Read the model definition and answer for the solid it produces. Units are mm, in the model's axes. A direction names the side the tool comes from. Coordinates: 2 decimals unless noted, no trailing zeros. Loops run counter-clockwise (first coordinate to the right, second up) from the corner with the lowest first, then second, coordinate; pieces in that order, holes last. Notation, with made-up numbers: M 29,31.25 L 83,31.25 A23 cw 83,49.25 Z; hole C 20.5,-28 d2. An arc over 180 degrees is marked long. Use one line per item in the form item = value. Start each with the question number.
1. The part is cut by section A-A (z = -20). Give the vertices of the cut face in (x, y).
2. For a pull along X with two mould halves and no side action, classify faces 1 (the conical face through (-86.28, -1.239, -12.833)), 2 (the conical face through (-65.93, 5.98, -7.72)), 3 (the flat face through (-58, 0, -40.287)) as released by +X, released by -X, zero draft, split by the parting line, or undercut.
3. Flat-ended cylindrical pins translate along their axes: pin 1 (12 mm diameter, centred on x = -53.5, y = 44.5, fed in from +Z); pin 2 (5 mm diameter, centred on y = -13.5, z = 14.5, fed in from +X); pin 3 (3 mm diameter, centred on x = -44, z = -13.5, fed in from -Y). Find the tip coordinate at first contact, or state that the pin passes through.
4. Find the intervals of material crossed by probe 1 along X at (y, z) = (-36.5, 19); probe 2 along X at (y, z) = (-6, 21.5); probe 3 along Y at (x, z) = (-81, 21), in increasing order. Write a range as [from, to].
5. The part is cut by section B-B (z = 21.5). Give the vertices of the cut face in (x, y).
6. A tool of negligible diameter and unlimited length cuts with its end or side. For faces 4 (the cylindrical face through (-83.5, -1.12, -27.41)), 5 (the conical face through (-107.31, 37.72, 29.41)), from which of +Z, -Z, +X, -X, +Y, -Y can it reach the whole face along a straight path? Write none if from no direction.
7. The part is cut by section C-C (z = 13). Give the vertices of the cut face in (x, y), plus the area to 3 significant figures.
from build123d import *

# Parameters (mm, degrees)
F2_R     = 25.4
F3_DEPTH = 25.4
F4_DEPTH = 76.2


with BuildPart() as f1:
    # F0 (on Front) → F1 (revolve)
    with BuildSketch(Plane.XZ):
        Polygon((-58.1262356877, -14.8871221304), (-58.1262356877, -40.2871221304), (-32.7262356877, -40.2871221304), (-32.7262356877, -14.8871221304), (11.7363044992, 17.9430041462), (3.4545188379, 29.9932819682), align=None)
    revolve(axis=Axis((-58.1262356877, 0, -27.5871221304), (0, 0, -1)))


with BuildPart() as f3:
    # F2 (on face) → F3 (new body)
    with BuildSketch(Plane(origin=(0, 0, -40.2871221304), x_dir=(1, 0, 0), z_dir=(0, 0, -1))):
        with Locations((-58.1262356877, 0)):
            Circle(F2_R)
    extrude(amount=F3_DEPTH)

    # F4 (cut): a face of the model
    f4_faces = [f3.faces().sort_by_distance(p)[0] for p in [
        (-58.1262356877, 0, -65.6871221304),
    ]]
    extrude(f4_faces, amount=-F4_DEPTH, mode=Mode.SUBTRACT)


solid = f1.part
Computed values:
q1.outline = C -58.13,0 d50.8
q2.face_1 = split by the parting line
q2.face_2 = undercut
q2.face_3 = zero draft
q3.pin_1 = 22.09
q3.pin_2 = 9.15
q3.pin_3 = -25.82
q4.probe_1 = [-116.84, -86.93], [-29.32, 0.59]
q4.probe_2 = [-125.28, -107.69], [-8.56, 9.02]
q4.probe_3 = [-63.78, -43.61], [43.61, 63.78]
q5.outline = C -58.13,0 d134.84; hole C -58.13,0 d99.85
q6.face_4 = -Z
q6.face_5 = +Z
q7.outline = C -58.13,0 d126.34; hole C -58.13,0 d76.53
q7.area = 7,940 mm²
